Autodesk Inventor part; units mm, degrees
ref_plane "YZ Plane" through (0, 0, 0) normal (1, 0, 0) x (0, 1, 0)
ref_plane "XZ Plane" through (0, 0, 0) normal (0, 1, 0) x (-1, 0, 0)
ref_plane "XY Plane" through (0, 0, 0) normal (0, 0, 1) x (1, 0, 0)
sketch "Skizze1" plane through (0, 0, 0) normal (0, 1, 0) x (-1, 0, 0)
  line L0 (0, 0) -> (60, 0)
  line L1 (60, 0) -> (60, 81.5)
  line L2 (60, 81.5) -> (60, 141.5)
  line L3 (60, 141.5) -> (0, 141.5)
  line L4 (0, 141.5) -> (0, 81.5)
  line L5 (0, 81.5) -> (60, 81.5)
  line L6 (0, 81.5) -> (0, 0)
  line L7 (60, 0) -> (0, 0)
  circle A0 centre (50, 116.5) radius 2.5
  circle A1 centre (50, 106.5) radius 2.5
  line L8 (0, 0) -> (-1.5, 0)
  line L9 (-1.5, 0) -> (-1.5, 141.5)
  line L10 (-1.5, 141.5) -> (0, 141.5)
  line L11 (0, 141.5) -> (0, 0)
  line L12 (-1.5, 141.5) -> (61.5, 141.5)
  line L13 (61.5, 141.5) -> (61.5, 143)
  line L14 (61.5, 143) -> (-1.5, 143)
  line L15 (-1.5, 143) -> (-1.5, 141.5)
  line L16 (61.5, 141.5) -> (60, 141.5)
  line L17 (60, 141.5) -> (60, 0)
  line L18 (60, 0) -> (61.5, 0)
  line L19 (61.5, 0) -> (61.5, 141.5)
  line L20 (61.5, 0) -> (-1.5, 0)
  line L21 (-1.5, 0) -> (-1.5, -1.5)
  line L22 (-1.5, -1.5) -> (61.5, -1.5)
  line L23 (61.5, -1.5) -> (61.5, 0)
  line L24 (61.5, 71.5) -> (61.5, 80)
  line L25 (61.5, 80) -> (-1.5, 80)
  line L26 (-1.5, 80) -> (-1.5, 70.75)
  line L27 (0, 141.5) -> (18, 141.5)
  line L28 (18, 141.5) -> (18, 131.5)
  line L29 (18, 131.5) -> (0, 131.5)
  line L30 (0, 131.5) -> (0, 141.5)
  line L31 (18, 131.5) -> (21.5, 131.5)
  line L32 (21.5, 131.5) -> (21.5, 141.5)
  line L33 (21.5, 141.5) -> (18, 141.5)
  line L34 (18, 141.5) -> (18, 131.5)
  line L35 (21.5, 131.5) -> (28.5, 131.5)
  line L36 (28.5, 131.5) -> (28.5, 141.5)
  line L37 (28.5, 141.5) -> (21.5, 141.5)
  line L38 (21.5, 141.5) -> (21.5, 131.5)
  line L39 (0, 81.5) -> (18, 81.5)
  line L40 (18, 81.5) -> (18, 91.5)
  line L41 (18, 91.5) -> (0, 91.5)
  line L42 (0, 91.5) -> (0, 81.5)
  line L43 (18, 81.5) -> (21.5, 81.5)
  line L44 (21.5, 81.5) -> (21.5, 91.5)
  line L45 (21.5, 91.5) -> (18, 91.5)
  line L46 (18, 91.5) -> (18, 81.5)
  line L47 (21.5, 81.5) -> (28.5, 81.5)
  line L48 (28.5, 81.5) -> (28.5, 91.5)
  line L49 (28.5, 91.5) -> (21.5, 91.5)
  line L50 (21.5, 91.5) -> (21.5, 81.5)
  line L51 (0, 116.5) -> (17, 116.5)
  line L52 (17, 116.5) -> (17, 106.5)
  line L53 (17, 106.5) -> (0, 106.5)
  line L54 (0, 106.5) -> (0, 116.5)
  line L55 (0, 75) -> (10, 75)
  line L56 (10, 75) -> (10, 71)
  line L57 (10, 71) -> (0, 71)
  line L58 (0, 71) -> (0, 75)
  line L59 (60, 71) -> (60, 73.5)
  line L60 (60, 5) -> (60, 9)
  line L61 (60, 75) -> (50, 75)
  line L62 (50, 75) -> (50, 71)
  line L63 (50, 71) -> (60, 71)
  line L64 (60, 71) -> (60, 75)
  line L65 (0, 5) -> (10, 5)
  line L66 (10, 5) -> (10, 9)
  line L67 (10, 9) -> (0, 9)
  line L68 (0, 9) -> (0, 5)
  line L69 (60, 5) -> (50, 5)
  line L70 (50, 5) -> (50, 9)
  line L71 (50, 9) -> (60, 9)
  line L72 (60, 9) -> (60, 5)
  point P0 (0, 131.5)
  point P1 (0, 116.5)
  point P2 (0, 106.5)
  point P3 (28.5, 141.5)
  point P4 (60, 80)
  point P5 (0, 80)
  point P6 (21.5, 141.5)
  point P7 (18, 141.5)
  point P8 (0, 71)
  point P9 (0, 9)
  dimension "d0" = 81.5
  dimension "d1" = 60
  dimension "d2" = 60
  dimension "d3" = 5
  dimension "d4" = 10
  dimension "d5" = 5
  dimension "d6" = 10
  dimension "d7" = 25
  dimension "d11" = 1.5
  dimension "d12" = 1.5
  dimension "d13" = 1.5
  dimension "d14" = 1.5
  dimension "d15" = 1.5
  dimension "d16" = 10
  dimension "d17" = 18
  dimension "d18" = 3.5
  dimension "d19" = 7
  dimension "d20" = 10
  dimension "d21" = 17
  dimension "d59" = 0
  dimension "d60" = 25
  dimension "d61" = 10
  dimension "d92" = 4
  dimension "d93" = 10
  dimension "d94" = 5
  dimension "d100" = 10
  dimension "d101" = 4
  dimension "d102" = 10
  dimension "d103" = 5
  dimension "d104" = 70
  dimension "d105" = 40
  dimension "d115" = 144.5
extrude "Extrusion1" add sketch "Skizze1" along normal blind 1.5 contours L6 L65 L66 L67 L57 L56 L55 L25 L1 L61 L62 L63 L71 L70 L69 L0 | L6 L67 L66 L65 | L69 L70 L71 L1 | L6 L55 L56 L57 | L63 L62 L61 L1 | L2 L5 L48 L49 L45 L41 L4 L53 L52 L51 L29 L31 L35 L36 L3
extrude "Extrusion2" add sketch "Skizze1" along normal blind 30 contours L3 L32 L31 L28 | L40 L45 L44 L5
extrude "Extrusion3" add sketch "Skizze1" along normal blind 35 contours L36 L35 L32 L3 | L5 L44 L49 L48
extrude "Extrusion4" add sketch "Skizze1" along normal blind 35 contours L3 L28 L29 L4 | L4 L41 L40 L5
extrude "Extrusion5" add sketch "Skizze1" along normal blind 25 contours L51 L52 L53 L4
extrude "Extrusion6" add sketch "Skizze1" along normal blind 60 contours L8 L9 L25 L6 | L0 L18 L23 L22 L21 L8 | L1 L25 L19 L18 | L9 L10 L4 L6 L25 | L25 L1 L2 L12 L19 | L15 L14 L13 L12 L3 L10 | L6 L5 L1 L25
sketch "Skizze3" plane through (0, 1.5, 80) normal (0, 0, -1) x (-1, 0, 0)
  point P0 (0, -1.5)
  point P1 (52.7194, 27.4431)
hole "Bohrung1" at (-52.7194, 28.9431, 80) direction (0, 0, 1) diameter 5 depth 2
sketch "Skizze4" plane through (-61.5, 0, -1.5) normal (-1, 0, 0) x (0, 0, 1)
  line L0 (0, 60) -> (144.5, 60)
  line L1 (0, 0) -> (0, 60)
  line L2 (144.5, 60) -> (0, 60)
  line L3 (0, 60) -> (0, 58)
  line L4 (0, 58) -> (144.5, 58)
  line L5 (144.5, 58) -> (144.5, 60)
  point P0 (1.5, 0)
  dimension "d41" = 2
extrude "Extrusion7" add sketch "Skizze4" along normal blind 1.5
sketch "Skizze5" plane through (1.5, 0, 143) normal (1, 0, 0) x (0, 0, -1)
  line L0 (0, 58) -> (0, 60)
  line L1 (0, 58) -> (144.5, 58)
  line L2 (0, 60) -> (144.5, 60)
  line L3 (144.5, 60) -> (144.5, 58)
  line L4 (144.5, 58) -> (0, 58)
  line L5 (0, 58) -> (0, 60)
  line L6 (144.5, 0) -> (144.5, 58)
  line L7 (0, 0) -> (144.5, 0)
  line L8 (144.5, 0) -> (144.5, 2)
  line L9 (0, 2) -> (0, 0)
  line L10 (0, 0) -> (0, 60)
  line L11 (0, 0) -> (10, 0)
  line L12 (10, 0) -> (10, 10)
  line L13 (10, 10) -> (0, 10)
  line L14 (0, 10) -> (0, 0)
  line L15 (144.5, 0) -> (134.5, 0)
  line L16 (134.5, 0) -> (134.5, 10)
  line L17 (134.5, 10) -> (144.5, 10)
  line L18 (144.5, 10) -> (144.5, 0)
  point P0 (143, 0)
  point P1 (134.5, 0)
  point P2 (0, 10)
  dimension "d44" = 2
  dimension "d48" = 10
  dimension "d49" = 10
  dimension "d50" = 10
  dimension "d51" = 10
extrude "Extrusion8" add sketch "Skizze5" along normal blind 1.5 contours L0 L2 L3 L1
extrude "Extrusion9" add sketch "Skizze5" along normal blind 3.5 contours L13 L12 L7 L9 L10 | L6 L7 L16 L17
sketch "Skizze6" plane through (-61.5, 0, -1.5) normal (0, 0, -1) x (-1, 0, 0)
  line L0 (1.5, 60) -> (1.5, 58)
  line L1 (-64.5, 58) -> (-64.5, 60)
  line L2 (0, 58) -> (1.5, 58)
  line L3 (1.5, 60) -> (-64.5, 60)
  line L4 (0, 0) -> (0, 58)
  line L5 (-63, 10) -> (-63, 58)
  line L6 (-66.5, 0) -> (-66.5, 10)
  point P0 (-61.5, 0)
  dimension "d54" = 66
  dimension "d55" = 2
  dimension "d56" = 63
  dimension "d57" = 3.5
sketch "Skizze7" plane through (-61.5, 0, -1.5) normal (0, 0, -1) x (-1, 0, 0)
  line L0 (-43.5, 48.5) -> (-46.5, 48.5)
  line L1 (-46.5, 48.5) -> (-46.5, 36.5)
  line L2 (-46.5, 36.5) -> (-43.5, 36.5)
  line L3 (-43.5, 36.5) -> (-43.5, 48.5)
  line L4 (-42, 50) -> (-48, 50)
  line L5 (-48, 50) -> (-48, 35)
  line L6 (-48, 35) -> (-42, 35)
  line L7 (-42, 35) -> (-42, 50)
  line L8 (-63, 10) -> (-63, 58)
  line L9 (1.5, 60) -> (-64.5, 60)
  circle A0 centre (-14.75, 42.5) radius 1.75
  line L10 (-11.5, 45.75) -> (-18, 45.75)
  line L11 (-18, 45.75) -> (-18, 39.25)
  line L12 (-18, 39.25) -> (-11.5, 39.25)
  line L13 (-11.5, 39.25) -> (-11.5, 45.75)
  line L14 (-10, 47.25) -> (-19.5, 47.25)
  line L15 (-19.5, 47.25) -> (-19.5, 37.75)
  line L16 (-19.5, 37.75) -> (-10, 37.75)
  line L17 (-10, 37.75) -> (-10, 47.25)
  line L18 (0, 0) -> (0, 58)
  line L19 (-61.5, 1.5) -> (-1.5, 1.5)
  point P0 (-61.5, 0)
  dimension "d62" = 3
  dimension "d63" = 12
  dimension "d64" = 1.5
  dimension "d65" = 1.5
  dimension "d66" = 1.5
  dimension "d67" = 1.5
  dimension "d68" = 15
  dimension "d69" = 10
  dimension "d70" = 3.5
  dimension "d71" = 17.5
  dimension "d72" = 3.25
  dimension "d73" = 3.25
  dimension "d74" = 6.5
  dimension "d75" = 6.5
  dimension "d76" = 1.5
  dimension "d77" = 1.5
  dimension "d78" = 1.5
  dimension "d79" = 1.5
  dimension "d80" = 10
  dimension "d91" = 33.5
  dimension "d108" = 58.5
extrude "Extrusion10" cut sketch "Skizze7" against normal blind 1.5 contours A0
extrude "Extrusion11" add sketch "Skizze7" against normal blind 3.5 contours L17 L16 L15 L14
extrude "Extrusion12" cut sketch "Skizze7" against normal blind 1.5 contours L3 L2 L1 L0
extrude "Extrusion13" add sketch "Skizze7" along normal blind 5 and the other way blind 6.5 contours L7 L6 L5 L4
extrude "Extrusion14" add sketch "Skizze1" along normal blind 10 contours L6 L55 L56 L57
extrude "Extrusion15" add sketch "Skizze1" along normal blind 10 contours L6 L67 L66 L65
extrude "Extrusion16" add sketch "Skizze1" along normal blind 10 contours L63 L62 L61 L1
extrude "Extrusion17" add sketch "Skizze1" along normal blind 10 contours L69 L70 L71 L1
properties part number "Box-Pumpe.v2"
Work out the finished part from the listing and answer in its coordinate system (mm). A direction names the side the tool comes from. Round coordinates to 2 decimals unless told otherwise and drop trailing zeros. Loops run counter-clockwise (first coordinate to the right, second up) from the corner with the lowest first, then second, coordinate; pieces in that order, holes last. Notation, with made-up numbers: (-38.5, 35.5) -> (-29.5, 35.5) arc R30 ccw to (-29.5, 73.5) -> close; hole circle Ø3 at (33, -2.5). An arc over 180 degrees is marked (long way). Write each question's results on one line, items separated by ' | '. Start each with the question number.
1. Find the intervals of material crossed by probe 1 along Z at (x, y) = (-50, 0.45); probe 2 along Z at (x, y) = (-52.5, 21); probe 3 along X at (y, z) = (6, 36.5), in increasing order. Write a range as from..to.
2. For a pull along X with two mould halves and no side action, classify faces 4 (the face through (5, 5, 4)), 5 (the face through (-61.5, 29, 70)), 6 (the face through (-9, 13, 106.5)), 7 (the face through (3, 5, 8.5)) as +X half, -X half, draft (parallel to the pull), parting line (faces both ways), or undercut.
3. Section A-A (y = 55) is taken. Determine the outline of the cut face in (x, z), plus the area to 4 significant figures.
4. Section B-B (x = -58) is taken. Determine the outline of the cut face in (y, z).
5. A tool of negligible diameter and unlimited length cuts with its end or side. For faces 1 (the face through (-16, 35, 3)), 2 (the face through (3, 10, 4)), 3 (the face through (-18, 32, 86)), from which of +Z, -Z, +X, -X, +Y, -Y can it reach the whole face along a straight path? Write none if from no direction.
6. Given pin 1 Ø8 at (x, z) = (-50, 116.5) entering from +Y; pin 2 Ø2 at (y, z) = (24, 31) entering from +X; pin 3 Ø8 at (x, z) = (-14.5, 93) entering from -Y; pin 4 Ø5 at (y, z) = (19, 54.5) entering from -X, each flat-ended and moving along its own axis, determine where each tip first touches the part or whether it passes through.
7. Section D-D (y = 23.5) is taken. Determine the outline of the cut face in (x, z).
8. Section C-C (y = 42.5) is taken. State how many separate pieces and enclosed holes the cut face has, plus the area to 3 significant figures.
Evaluation:
1) probe 1: z = -1.5..104, 109..114, 119..143 | probe 2: z = -1.5..0, 80..81.5, 141.5..143 | probe 3: x = -61.5..-60, 0..1.5
2) face 4: +X half | face 5: -X half | face 6: undercut | face 7: draft
3) outline: (-61.5, -1.5) -> (1.5, -1.5) -> (1.5, 143) -> (-61.5, 143) -> close; hole (-60, 0) -> (0, 0) -> (0, 80) -> (-60, 80) -> close; hole (-60, 81.5) -> (0, 81.5) -> (0, 141.5) -> (-60, 141.5) -> close | area: 703.5 mm2
4) outline: (0, -1.5) -> (60, -1.5) -> (60, 0) -> (1.5, 0) -> (1.5, 5) -> (10, 5) -> (10, 9) -> (1.5, 9) -> (1.5, 71) -> (10, 71) -> (10, 75) -> (1.5, 75) -> (1.5, 80) -> (60, 80) -> (60, 81.5) -> (1.5, 81.5) -> (1.5, 141.5) -> (60, 141.5) -> (60, 143) -> (0, 143) -> close
5) face 1: none | face 2: +Z, -Z, +X | face 3: +Y
6) pin 1: stops at y = 1.5 | pin 2: stops at x = 1.5 | pin 3: stops at y = 0 | pin 4: stops at x = -61.5
7) outline: (-61.5, -1.5) -> (1.5, -1.5) -> (1.5, 143) -> (-61.5, 143) -> close; hole (-60, 0) -> (0, 0) -> (0, 80) -> (-60, 80) -> close; hole (-60, 81.5) -> (-28.5, 81.5) -> (-28.5, 91.5) -> (0, 91.5) -> (0, 106.5) -> (-17, 106.5) -> (-17, 116.5) -> (0, 116.5) -> (0, 131.5) -> (-28.5, 131.5) -> (-28.5, 141.5) -> (-60, 141.5) -> close
8) separate pieces: 2 | enclosed holes: 1 | area: 730 mm2
